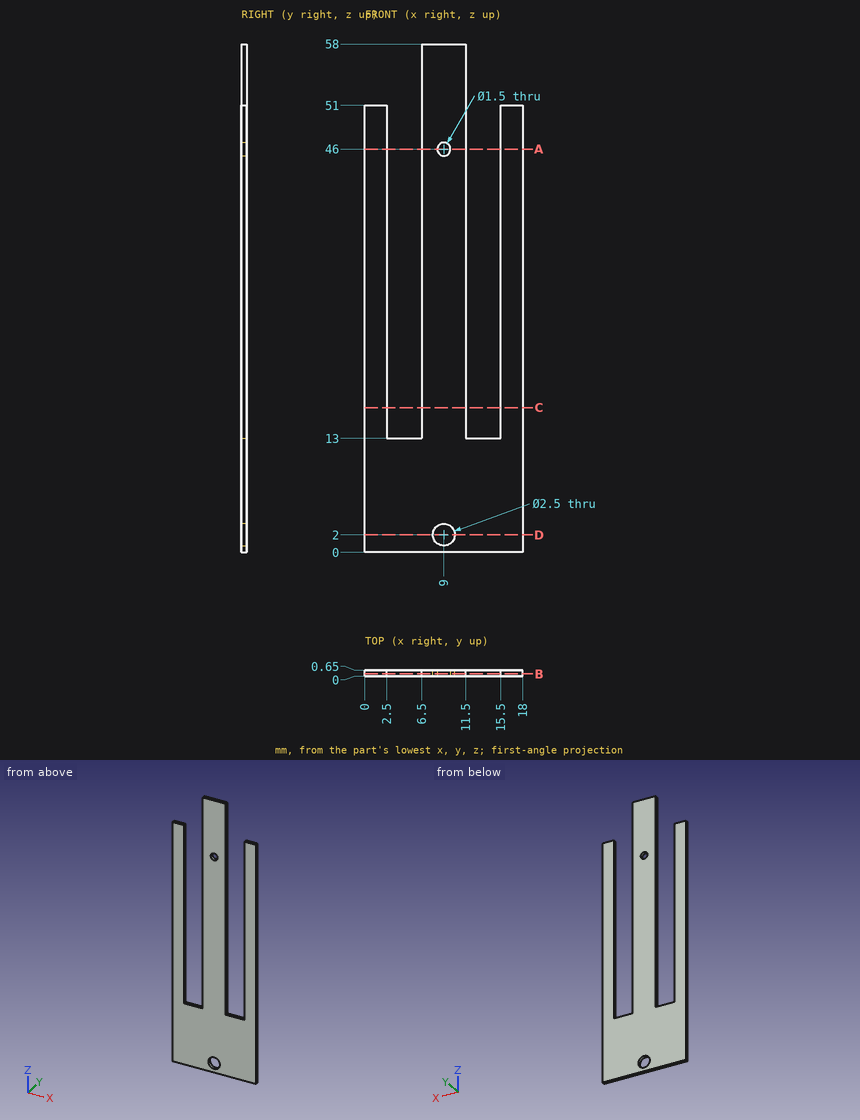
Verification items for this drawing (mm, ordinates from the low corner). Coordinates: 2 decimals unless noted, no trailing zeros. Loops run counter-clockwise (first coordinate to the right, second up) from the corner with the lowest first, then second, coordinate; pieces in that order, holes last. Notation, with made-up numbers: (33, 69.25) -> (68, 69.25) arc R16 cw to (68, 100.25) -> close; hole circle Ø10 at (-15.75, -15.75). An arc over 180 degrees is marked (long way). Answer in a Markdown table with one row per item. Add a question column.
1. Section check B-B, the plane y = 0.25. Enter the section's corners in (x, z).
2. Depth check by flat-ended pin: P1, Ø2, axis at x = 9, z = 2, coming from the +Y side. Enter the tip coordinate at first touch or a pass-through.
3. Section check D-D, the plane z = 2. Enter the section's corners in (x, y).
4. Section check C-C, the plane z = 16.5. Enter the section's corners in (x, y), then the cut area to 3 significant figures.
5. Material ranges on probe 1 along X at (y, z) = (0.35, 46); probe 2 along X at (y, z) = (0.45, 38.5); probe 3 along Z at (x, y) = (9.25, 0.3), recorded low to high. Write a range as [from, to].
6. Section check A-A, the plane z = 46. Enter the section's corners in (x, y).
Derived:
| question | item | result |
|---|---|---|
| 1 | outline | (0, 0) -> (18, 0) -> (18, 51) -> (15.5, 51) -> (15.5, 13) -> (11.5, 13) -> (11.5, 58) -> (6.5, 58) -> (6.5, 13) -> (2.5, 13) -> (2.5, 51) -> (0, 51) -> close; hole circle Ø2.5 at (9, 2); hole circle Ø1.5 at (9, 46) |
| 2 | P1 | passes through |
| 3 | outline | (0, 0) -> (7.75, 0) -> (7.75, 0.65) -> (0, 0.65) -> close; (10.25, 0) -> (18, 0) -> (18, 0.65) -> (10.25, 0.65) -> close |
| 4 | outline | (0, 0) -> (2.5, 0) -> (2.5, 0.65) -> (0, 0.65) -> close; (6.5, 0) -> (11.5, 0) -> (11.5, 0.65) -> (6.5, 0.65) -> close; (15.5, 0) -> (18, 0) -> (18, 0.65) -> (15.5, 0.65) -> close |
| 4 | area | 6.50 mm² |
| 5 | probe 1 | x = [0, 2.5], [6.5, 8.25], [9.75, 11.5], [15.5, 18] |
| 5 | probe 2 | x = [0, 2.5], [6.5, 11.5], [15.5, 18] |
| 5 | probe 3 | z = [0, 0.78], [3.22, 45.29], [46.71, 58] |
| 6 | outline | (0, 0) -> (2.5, 0) -> (2.5, 0.65) -> (0, 0.65) -> close; (6.5, 0) -> (8.25, 0) -> (8.25, 0.65) -> (6.5, 0.65) -> close; (9.75, 0) -> (11.5, 0) -> (11.5, 0.65) -> (9.75, 0.65) -> close; (15.5, 0) -> (18, 0) -> (18, 0.65) -> (15.5, 0.65) -> close |
